Can you work these out from the model? Positions are in its coordinate system, mm. Face numbers are marked on the shaded views. A direction names the side the tool comes from. Coordinates: 2 decimals unless noted, no trailing zeros. Order: outer loops, then holes, each group sorted by start corner. A loop starts at its lowest first (then second) coordinate and runs counter-clockwise, first axis right, second up. Notation, with made-up numbers: (-12, 18.25) - (8, 18.25) arc R24 ccw to (8, 53.25) - close; hole circle Ø6 at (-10, 62.5). An arc over 180 degrees is marked (long way). Use a Markdown table: item, result. Add a question column.
(1) If I drill on L1, parallel to Y at x = 0, z = 4.75; L2, parallel to Y at x = 0.25, z = 8.5; L3, parallel to X at y = -0.5, z = 5.5, over which ranges is the centre line in solid material (lowest first)? Write a range as [from, to].
(2) I want a section at B-B (y = 5.06). List the corners of the cut face in (x, z) for me, and give its area (3 significant figures).
(3) On a 3-axis mill with a long thin cutter (end or side, diameter ignored), from which of +Z, -Z, +X, -X, +Y, -Y can I reach the whole of each face in a straight line? I mean the marked faces 1 and 2. Say none if no direction works.
(4) I want a section at C-C (z = 6.5). List the corners of the cut face in (x, y) for me.
(5) I want a section at D-D (x = -3.5). List the corners of the cut face in (y, z) for me.
(6) For pin 1 Ø5.5 at (x, z) = (-0.5, 10.5) entering from -Y, with a flat end and sliding along its axis, tell me the tip position at first contact or that it passes through.
(7) I want a section at A-A (x = 0). List the corners of the cut face in (y, z) for me.
```python
from build123d import *

# Parameters (mm, degrees)
F0_W     = 23.1
F0_H     = 36.12
F2_DEPTH = 7.7
F1_W     = 23.1
F1_H     = 26
F3_DEPTH = 12.6
F4_R     = 6.64
F5_DEPTH = 12.6


with BuildPart() as f2:
    # F0 (on Top) → F2 (new body)
    with BuildSketch(Plane.XY):
        Rectangle(F0_W, F0_H)
    extrude(amount=F2_DEPTH)

    # F1 (on Top) → F3 (join)
    with BuildSketch(Plane.XY):
        with Locations((0, 5.06)):
            Rectangle(F1_W, F1_H)
    extrude(amount=F3_DEPTH)

    # F4 (on Top) → F5 (cut)
    with BuildSketch(Plane.XY):
        with Locations((0, 5.06)):
            Circle(F4_R)
    extrude(amount=F5_DEPTH, mode=Mode.SUBTRACT)


solid = f2.part
```
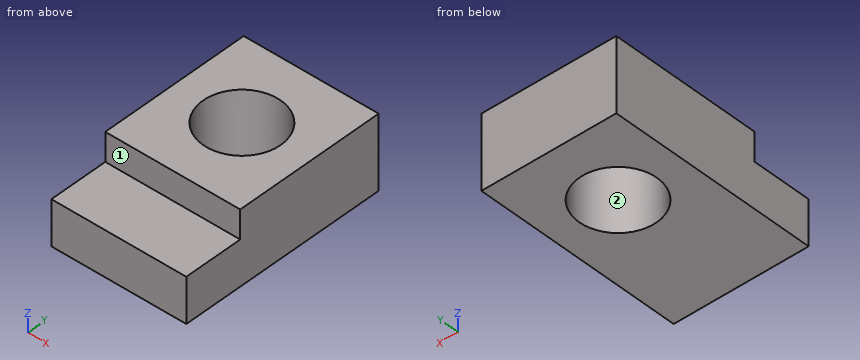
Answers follow:
| question | item | result |
|---|---|---|
| 1 | L1 | y = [-18.06, -1.58], [11.7, 18.06] |
| 1 | L2 | y = [-7.94, -1.58], [11.7, 18.06] |
| 1 | L3 | x = [-11.55, -3.63], [3.63, 11.55] |
| 2 | outline | (-11.55, 0) - (-6.64, 0) - (-6.64, 12.6) - (-11.55, 12.6) - close; (6.64, 0) - (11.55, 0) - (11.55, 12.6) - (6.64, 12.6) - close |
| 2 | area | 124 mm² |
| 3 | face 1 | +Z, +X, -X, -Y |
| 3 | face 2 | +Z, -Z |
| 4 | outline | (-11.55, -18.06) - (11.55, -18.06) - (11.55, 18.06) - (-11.55, 18.06) - close; hole circle Ø13.28 at (0, 5.06) |
| 5 | outline | (-18.06, 0) - (-0.58, 0) - (-0.58, 12.6) - (-7.94, 12.6) - (-7.94, 7.7) - (-18.06, 7.7) - close; (10.7, 0) - (18.06, 0) - (18.06, 12.6) - (10.7, 12.6) - close |
| 6 | pin 1 | stops at y = -7.94 |
| 7 | outline | (-18.06, 0) - (-1.58, 0) - (-1.58, 12.6) - (-7.94, 12.6) - (-7.94, 7.7) - (-18.06, 7.7) - close; (11.7, 0) - (18.06, 0) - (18.06, 12.6) - (11.7, 12.6) - close |
